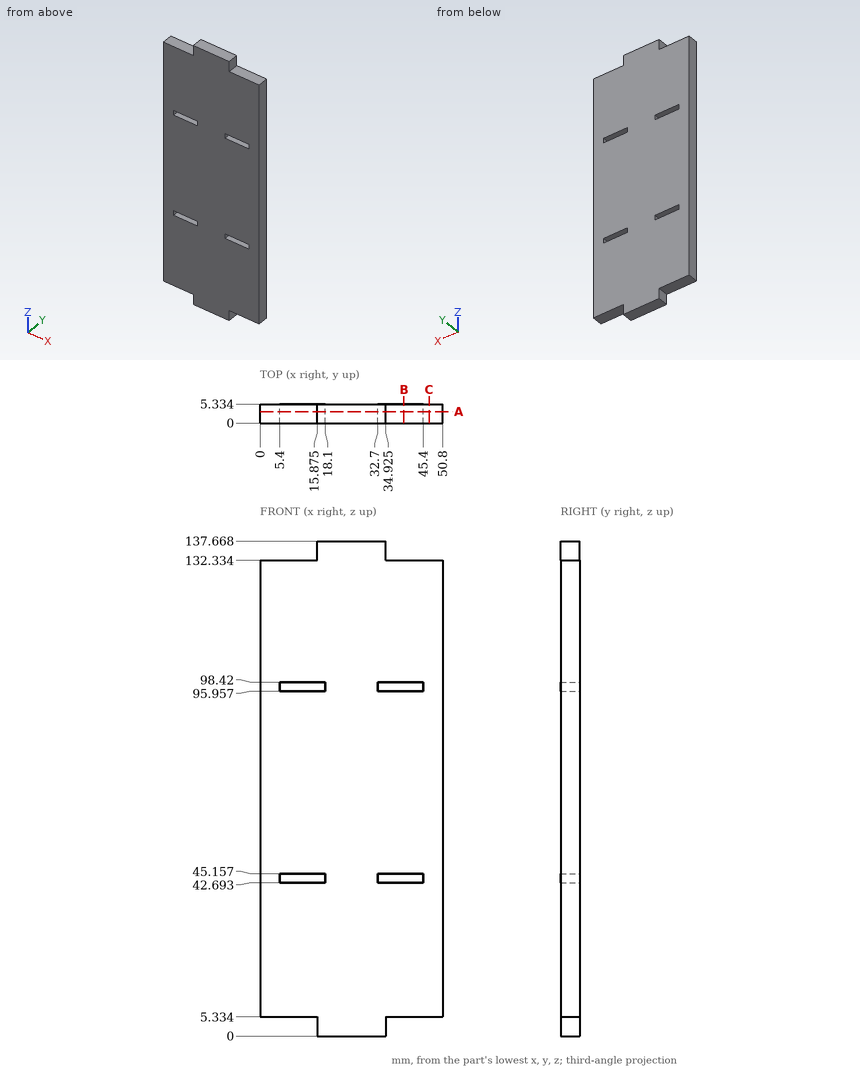
Source: three-view drawing plus pictorial views. Frame: mm from the lowest corner of the part. Coordinates: 2 decimals unless noted, no trailing zeros. Order: outer loops, then holes, each group sorted by start corner. A loop starts at its lowest first (then second) coordinate and runs counter-clockwise, first axis right, second up. Notation, with made-up numbers: M -17,30 L -13,30 A7 cw -13,36 Z; hole C 67.25,-37.75 d9. An arc over 180 degrees is marked long. One line per question, with ' | ' between items.
Item 1: Section B-B (x = 40). Output: boundary loops of the cut face in (y, z), then the cut area to 3 significant figures.
Geometry results:
outline: M 0,5.33 L 5.33,5.33 L 5.33,42.69 L 0,42.69 Z; M 0,45.16 L 5.33,45.16 L 5.33,95.96 L 0,95.96 Z; M 0,98.42 L 5.33,98.42 L 5.33,132.33 L 0,132.33 Z | area: 651 mm^2
Item 2: Pin query (flat end, axial travel): pin 1 (2.5 mm diameter, centred on y = 2.5, z = 44.5, fed in from -X); pin 2 (1.6 mm diameter, centred on x = 42, y = 3, fed in from +Z); pin 3 (2.5 mm diameter, centred on x = 10.5, y = 2, fed in from -Z). Return the tip coordinate at first contact, or that it passes through.
Geometry results:
pin 1: stops at x = 0 | pin 2: stops at z = 132.33 | pin 3: stops at z = 5.33
Item 3: Section A-A (y = 3.2). Output: boundary loops of the cut face in (x, z) (1 decimal), then the cut area to 3 significant figures.
Geometry results:
outline: M 0,5.3 L 15.9,5.3 L 15.9,0 L 34.9,0 L 34.9,5.3 L 50.8,5.3 L 50.8,132.3 L 34.9,132.3 L 34.9,137.7 L 15.9,137.7 L 15.9,132.3 L 0,132.3 Z; hole M 5.4,42.7 L 18.1,42.7 L 18.1,45.2 L 5.4,45.2 Z; hole M 5.4,96 L 18.1,96 L 18.1,98.4 L 5.4,98.4 Z; hole M 32.7,42.7 L 45.4,42.7 L 45.4,45.2 L 32.7,45.2 Z; hole M 32.7,96 L 45.4,96 L 45.4,98.4 L 32.7,98.4 Z | area: 6,530 mm^2
Item 4: Section C-C (x = 47). Output: boundary loops of the cut face in (y, z).
Geometry results:
outline: M 0,5.33 L 5.33,5.33 L 5.33,132.33 L 0,132.33 Z
Item 5: Ray query, line 1 along Z through (x, y) = (11.5, 2); line 2 along X through (y, z) = (4.4, 96); line 3 along Z through (x, y) = (34, 2.45). Return the intervals inside material, ascending.
Geometry results:
line 1: z = 5.33 to 42.69, 45.16 to 95.96, 98.42 to 132.33 | line 2: x = 0 to 5.4, 18.1 to 32.7, 45.4 to 50.8 | line 3: z = 0 to 42.69, 45.16 to 95.96, 98.42 to 137.67
